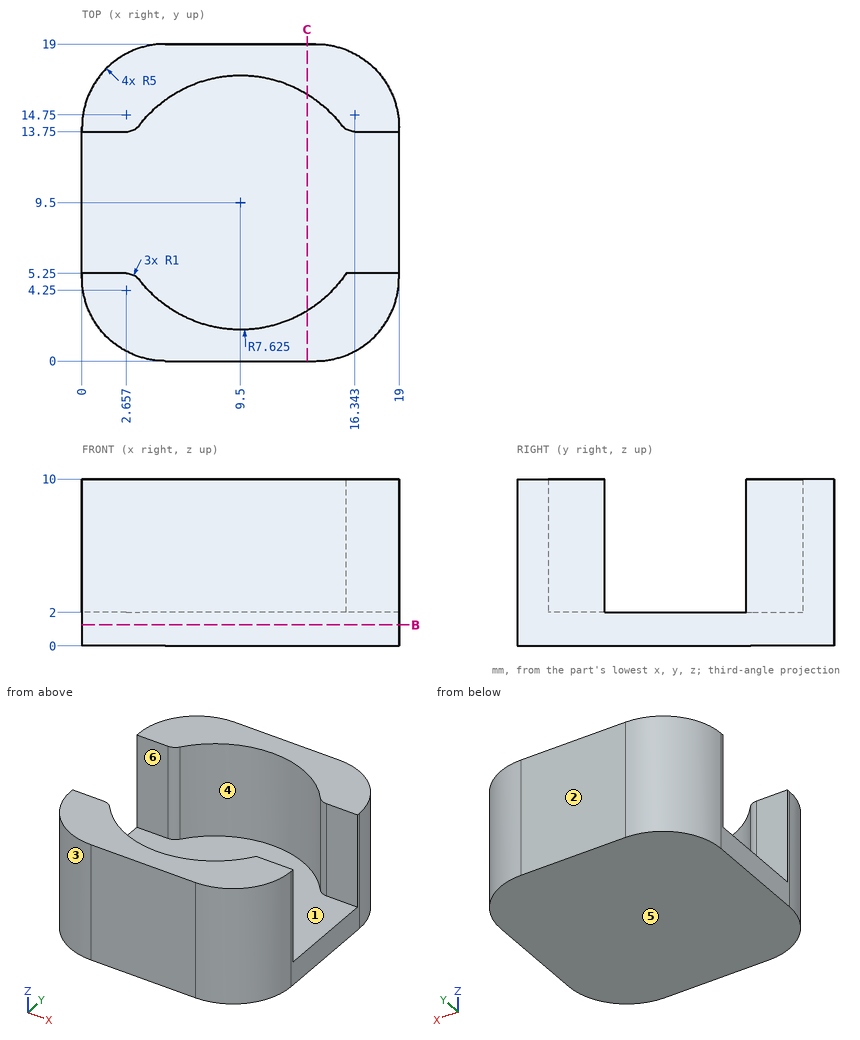
Geometry check sheet. Reference: drawing and pictorial views, mm from the part's lowest x, y, z. A direction names the side the tool comes from. Give positions to 0.01 mm unless a question says otherwise; leave off trailing zeros. Loops run counter-clockwise (first coordinate to the right, second up) from the corner with the lowest first, then second, coordinate; pieces in that order, holes last. Notation, with made-up numbers: (54, 66) -> (91, 66) arc R19 cw to (91, 89) -> close; hole circle Ø4 at (-30.5, 59). An arc over 180 degrees is marked (long way). Answer in a Markdown table with one row per item. Add a question column.
1) Gauge pin test, flat ends, axial feed: P1, Ø0.8, axis at x = 1, z = 4, coming from the -Y side; P2, Ø4.5, axis at x = 8, y = 12.5, coming from the +Z side; P3, Ø2.5, axis at x = 18, z = 7, coming from the +Y side. Record the tip position at first contact, or that the pin passes through.
2) Draft check along X on the marked faces 1, 2 and 3. Enter one of: pulls with the +X half, pulls with the -X half, needs draft (parallel to the pull), parting line crosses it, or undercut.
3) Material ranges on probe 1 along Z at (x, y) = (7.5, 3.5); probe 2 along X at (y, z) = (4.75, 0.5); probe 3 along X at (y, z) = (4.25, 7.25), recorded low to high. Write a range as from..to.
4) Cross-section at C-C on x = 13.5. Record the boundary of the cut face in (y, z).
5) Cross-section at B-B on z = 1.25. Record the boundary of the cut face in (x, y).
6) Set-up check for the marked faces 4, 5 and 6: record each of +Z, -Z, +X, -X, +Y, -Y from which the full face is reachable in a straight line by a thin tool's end or side.
Outcome:
| question | item | result |
|---|---|---|
| 1 | P1 | stops at y = 1.53 |
| 1 | P2 | stops at z = 2 |
| 1 | P3 | stops at y = 18.18 |
| 2 | face 1 | undercut |
| 2 | face 2 | needs draft |
| 2 | face 3 | pulls with the -X half |
| 3 | probe 1 | z = 0..2 |
| 3 | probe 2 | x = 0.01..18.99 |
| 3 | probe 3 | x = 0.06..3.97, 15.03..18.94 |
| 4 | outline | (0, 0) -> (19, 0) -> (19, 10) -> (15.99, 10) -> (15.99, 2) -> (3.01, 2) -> (3.01, 10) -> (0, 10) -> close |
| 5 | outline | (0, 5) arc R5 ccw to (5, 0) -> (14, 0) arc R5 ccw to (19, 5) -> (19, 14) arc R5 ccw to (14, 19) -> (5, 19) arc R5 ccw to (0, 14) -> close |
| 6 | face 4 | +Z |
| 6 | face 5 | -Z, +X, -X, +Y, -Y |
| 6 | face 6 | +Z, +X, -X |
